Input: part model. Units: mm. Frame: model coordinates. Coordinates: 2 decimals unless noted, no trailing zeros. Loops run counter-clockwise (first coordinate to the right, second up) from the corner with the lowest first, then second, coordinate; pieces in that order, holes last. Notation, with made-up numbers: (-32, 42) -> (14, 42) arc R22 cw to (14, 72) -> close; hole circle Ø9 at (-23, 42.5). An arc over 180 degrees is marked (long way). Answer as a JSON object with one key per item and string values.
from build123d import *

# Parameters (mm, degrees)
F0_R     = 9.525
F0_R_2   = 3.175
F1_DEPTH = 38.8874
F2_SIZE2 = 1.5748
F2_SIZE  = 1.5748
F3_SIZE2 = 1.5748
F3_SIZE  = 1.5748
F4_R     = 2.3749
F5_DEPTH = 12.7


with BuildPart() as f1:
    # F0 (on Right) → F1 (new body, symmetric)
    with BuildSketch(Plane.YZ):
        Circle(F0_R)
        Circle(F0_R_2, mode=Mode.SUBTRACT)
    extrude(amount=F1_DEPTH, both=True)

    # F2
    f2_edges = [f1.edges().sort_by_distance(p)[0] for p in [
        (38.8874, -9.525, 0),
    ]]
    chamfer(f2_edges, length=F2_SIZE, length2=F2_SIZE2)

    # F3
    f3_edges = [f1.edges().sort_by_distance(p)[0] for p in [
        (-38.8874, -9.525, 0),
    ]]
    chamfer(f3_edges, length=F3_SIZE, length2=F3_SIZE2)

    # F4 (on Front) → F5 (cut, symmetric)
    with BuildSketch(Plane.XZ):
        with Locations((26.1874, 0)):
            Circle(F4_R)
    extrude(amount=F5_DEPTH, both=True, mode=Mode.SUBTRACT)


solid = f1.part
1. Section query C-C (x = -32.5). Return loops of the section in (y, z) (3 decimals).
Reply:
{"outline": "circle Ø19.05 at (0, 0); hole circle Ø6.35 at (0, 0)"}
2. Mould query, pull axis X, two halves, no side actions, for faces 1 (the face through (38.887, 3.4, 0.1)), 2 (the face through (28.453, -5.868, 0.713)), 3 (the face through (-38.887, 3.4, 0.1)). Classes: pulls with the +X half, pulls with the -X half, needs draft (parallel to the pull), parting line crosses it, or undercut.
Reply:
{"face 1": "pulls with the +X half", "face 2": "undercut", "face 3": "pulls with the -X half"}
3. Section query B-B (z = 0). Return loops of the section in (x, y) (1 decimal).
Reply:
{"outline": "(-38.9, -8) -> (-37.3, -9.5) -> (23.8, -9.5) -> (23.8, -3.2) -> (-38.9, -3.2) -> close; (-38.9, 3.2) -> (23.8, 3.2) -> (23.8, 9.5) -> (-37.3, 9.5) -> (-38.9, 8) -> close; (28.6, -9.5) -> (37.3, -9.5) -> (38.9, -8) -> (38.9, -3.2) -> (28.6, -3.2) -> close; (28.6, 3.2) -> (38.9, 3.2) -> (38.9, 8) -> (37.3, 9.5) -> (28.6, 9.5) -> close"}
4. Pin query (flat end, axial travel): P1, Ø10, axis at x = 9, y = 6.5, coming from the -Z side; P2, Ø1, axis at x = -24, y = -6.5, coming from the -Z side; P3, Ø2, axis at x = 7.5, z = -3.5, coming from the -Y side; P4, Ø4, axis at x = 26.19, z = 0, coming from the -Y side. Return the tip coordinate at first contact, or that it passes through.
Reply:
{"P1": "stops at z = -9.41", "P2": "stops at z = -7.4", "P3": "stops at y = -9.19", "P4": "passes through"}
5. Line query: line 1 along Z through (x, y) = (21.5, 0) (3 decimals); line 2 along X through (y, z) = (3.75, 1.5). Output: solid intervals per line, ascending.
Reply:
{"line 1": "z = -9.525 to -3.175, 3.175 to 9.525", "line 2": "x = -38.89 to 24.35, 28.03 to 38.89"}
6. Section query A-A (y = 0). Return loops of the section in (x, z) (3 decimals).
Reply:
{"outline": "(-38.887, -7.95) -> (-37.313, -9.525) -> (37.313, -9.525) -> (38.887, -7.95) -> (38.887, -3.175) -> (-38.887, -3.175) -> close; (-38.887, 3.175) -> (38.887, 3.175) -> (38.887, 7.95) -> (37.313, 9.525) -> (-37.313, 9.525) -> (-38.887, 7.95) -> close"}
